Autodesk Inventor part; units mm, degrees
ref_plane "YZ Plane" through (0, 0, 0) normal (1, 0, 0) x (0, 1, 0)
ref_plane "XZ Plane" through (0, 0, 0) normal (0, 1, 0) x (-1, 0, 0)
ref_plane "XY Plane" through (0, 0, 0) normal (0, 0, 1) x (1, 0, 0)
sketch "Sketch1" plane through (0, 0, 0) normal (0, 0, 1) x (1, 0, 0)
  line L0 (0, 0) -> (0, 50.8)
  line L1 (0, 50.8) -> (3.175, 50.8)
  line L2 (3.175, 50.8) -> (3.175, 3.175)
  line L3 (3.175, 3.175) -> (123.825, 3.175)
  line L4 (123.825, 3.175) -> (123.825, 50.8)
  line L5 (123.825, 50.8) -> (127, 50.8)
  line L6 (127, 50.8) -> (127, 0)
  line L7 (127, 0) -> (0, 0)
  dimension "d0" = 3.175
  dimension "d2" = 3.175
  dimension "d3" = 3.175
  dimension "d4" = 127
  dimension "d5" = 50.8
extrude "Extrusion1" add sketch "Sketch1" along normal blind 50.8
sketch "Sketch2" plane through (127, 0, 0) normal (1, 0, 0) x (0, 0, -1)
  line L0 (0, 50.8) -> (0, 0)
  line L1 (0, 50.8) -> (-50.8, 50.8)
  line L2 (-50.8, 0) -> (-50.8, 50.8)
  line L3 (0, 0) -> (-50.8, 0)
  point P0 (0, 0)
  point P1 (-25.4, 22.225)
  dimension "d8" = 25.4
  dimension "d9" = 25.4
  dimension "d10" = 22.225
hole "Hole1" at (127, 22.225, 25.4) direction (-1, 0, 0) diameter 6.35 end through all
equation "\"d2\" = d0"
equation "\"d3\" = d0"
properties part number "ScissorLIftBracketOutside"
CAD build for the part. Positions are in the model's coordinates, mm. A direction names the side the tool comes from. Give positions to 0.01 mm unless a question says otherwise; leave off trailing zeros. Loops run counter-clockwise (first coordinate to the right, second up) from the corner with the lowest first, then second, coordinate; pieces in that order, holes last. Notation, with made-up numbers: M 76.25,89 L 110.25,89 A32 ccw 110.25,127 Z; hole C 70.25,-3.75 d6. An arc over 180 degrees is marked long. Answer in a Markdown table with one row per item. Add a question column.
Item 1: Tool access for faces 4 (the face through (63, 3, 0)), 5 (the face through (123.825, 27, 25)): list every direction of +Z, -Z, +X, -X, +Y, -Y with a clear straight run to the whole face (end or side of a thin tool).
Item 2: Probe probe 1 along Y at (x, z) = (2.05, 25.4); probe 2 along X at (y, z) = (12.5, 6) (3 decimals); probe 3 along Y at (x, z) = (97, 14) (3 decimals). List the from-to ranges inside material, lowest first.
Item 3: Mould opens along X. For faces 1 (the face through (0, 31, 25)), 2 (the face through (64, 0, 25)), 3 (the face through (63, 3.175, 25)) say: +X half, -X half, draft (parallel to the pull), parting line (faces both ways), or undercut.
Item 4: Band-saw the part on A-A on z = 25.4. Give the cut face in (x, y) (3 decimals).
Item 5: Band-saw the part on C-C on z = 18. Give the cut face in (x, y) (3 decimals).
Item 6: Band-saw the part on B-B on y = 17.5. Give the cut face in (x, z) (3 decimals).
Item 7: Drop flat-ended pins along their axis: P1, Ø12, axis at x = 32.5, y = 11.5, coming from the +Z side; P2, Ø4, axis at x = 71, z = 21.5, coming from the +Y side (3 decimals). Give the stop position or say it passes through.
Item 8: Band-saw the part on D-D on x = 113. Give the cut face in (y, z) (3 decimals), then the cut area to 3 significant figures.
Reply:
| question | item | result |
|---|---|---|
| 1 | face 4 | -Z, +X, -X, +Y, -Y |
| 1 | face 5 | +Z, -Z, +Y |
| 2 | probe 1 | y = 0 to 19.05, 25.4 to 50.8 |
| 2 | probe 2 | x = 0 to 3.175, 123.825 to 127 |
| 2 | probe 3 | y = 0 to 3.175 |
| 3 | face 1 | -X half |
| 3 | face 2 | draft |
| 3 | face 3 | undercut |
| 4 | outline | M 0,0 L 127,0 L 127,19.05 L 123.825,19.05 L 123.825,3.175 L 3.175,3.175 L 3.175,19.05 L 0,19.05 Z; M 0,25.4 L 3.175,25.4 L 3.175,50.8 L 0,50.8 Z; M 123.825,25.4 L 127,25.4 L 127,50.8 L 123.825,50.8 Z |
| 5 | outline | M 0,0 L 127,0 L 127,50.8 L 123.825,50.8 L 123.825,3.175 L 3.175,3.175 L 3.175,50.8 L 0,50.8 Z |
| 6 | outline | M 0,0 L 3.175,0 L 3.175,50.8 L 0,50.8 Z; M 123.825,0 L 127,0 L 127,50.8 L 123.825,50.8 Z |
| 7 | P1 | passes through |
| 7 | P2 | stops at y = 3.175 |
| 8 | outline | M 0,0 L 3.175,0 L 3.175,50.8 L 0,50.8 Z |
| 8 | area | 161 mm^2 |
